Autodesk Inventor part; units mm, degrees
ref_plane "YZ Plane" through (0, 0, 0) normal (1, 0, 0) x (0, 1, 0)
ref_plane "XZ Plane" through (0, 0, 0) normal (0, 1, 0) x (-1, 0, 0)
ref_plane "XY Plane" through (0, 0, 0) normal (0, 0, 1) x (1, 0, 0)
sketch "Sketch1" plane through (0, 0, 0) normal (0, 1, 0) x (-1, 0, 0)
  line L0 (14, 0) -> (0, 0)
  line L1 (0, 0) -> (0, -35.7)
  line L2 (0, -35.7) -> (14, -35.7)
  line L3 (14, -35.7) -> (14, 0)
  circle A0 centre (7, -7) radius 3.25
  circle A1 centre (7, -28.7) radius 3.25
  arc A2 (14, -7) -> (0, -7) centre (7, -7) ccw
  line L4 (14, -35.7) -> (14, -40.7)
  line L5 (14, -40.7) -> (8.75, -40.7)
  line L6 (5.25, -40.7) -> (0, -40.7)
  line L7 (0, -40.7) -> (0, -35.7)
  line L8 (8.75, -40.7) -> (5.25, -40.7)
  line L9 (14, -40.7) -> (46.5741, -73.2741)
  line L10 (46.5741, -73.2741) -> (55.0594, -64.7888)
  line L11 (55.0594, -64.7888) -> (14, -23.7294)
  circle A3 centre (7, -28.7) radius 7
  line L12 (14, -40.7) -> (3.5544, -34.7933)
  point P0 (7, -35.7)
  point P1 (11.375, -40.7)
  point P2 (7, 0)
  point P3 (0, -28.7)
  dimension "d0" = 6.5
  dimension "d1" = 21.7
  dimension "d2" = 7
  dimension "d3" = 7
  dimension "d4" = 14
  dimension "d9" = 5
  dimension "d20" = 12
  dimension "d21" = 135
extrude "Extrusion1" add sketch "Sketch1" along normal blind 4 contours L3 A2 L0 | A2 L1 L0 | A2 L3 A3 L1 | L11 L10 L9 L4 L3 | A3 | L3 L2 A3 | A3 L2 L12 | L4 L12 L2
fillet "Fillet1" radius 5 1 edges at (-14, 2, -40.7)
sketch "Sketch3" plane through (0, 4, 0) normal (0, 1, 0) x (1, 0, 0)
  line L0 (-14, 0) -> (0, 0)
  line L1 (0, 0) -> (0, 28.7)
  arc A0 (0, 28.7) -> (-3.5544, 34.7933) centre (-7, 28.7) ccw
  line L2 (-3.5544, 34.7933) -> (-13.4072, 40.3648)
  arc A1 (-14.4816, 41.1816) -> (-13.4072, 40.3648) centre (-10.946, 44.7171) ccw
  line L3 (-14.4816, 41.1816) -> (-46.5741, 73.2741)
  line L4 (-46.5741, 73.2741) -> (-55.0594, 64.7888)
  line L5 (-55.0594, 64.7888) -> (-14, 23.7294)
  line L6 (-14, 23.7294) -> (-14, 0)
  circle A2 centre (-7, 7) radius 3.25
  circle A3 centre (-7, 28.7) radius 3.25
  circle A4 centre (-7, 28.7) radius 7
  line L7 (-14, 23.7294) -> (-9.3072, 22.0912)
  line L8 (-14, 23.7294) -> (-14, 28.7)
  line L9 (-14.4816, 41.1816) -> (-21.444, 48.144)
  circle A5 centre (-7, 28.7) radius 12.5
  arc A6 (-15.8366, 37.541) -> (-14.4816, 41.1816) centre (-19.1353, 40.8413) ccw
  point P0 (-3.5544, 34.7933)
  point P1 (-11.499, 34.0628)
  point P2 (-3.5544, 34.7933)
  point P3 (-19.4892, 29.2187)
  point P4 (-15.8366, 37.541)
  point P5 (-14.1011, 40.8383)
  point P6 (0, 18.3438)
  point P7 (-12.5691, 39.8909)
  point P8 (-14, 18.3438)
  dimension "d24" = 25
extrude "Extrusion4" add sketch "Sketch3" along normal blind 2.5 contours L5 L4 L3 A6 A5
mirror "Mirror3" about plane through (-34.7643, 6.5, -51.2464) normal (0, 1, 0) of "Extrusion4", "Fillet1", "Extrusion1"
fillet "Fillet3" radius 7 4 edges at (0, 11, 0) (-14, 11, 0) (-14, 2, 0) (0, 2, 0)
properties part number "R2_3DPrint"
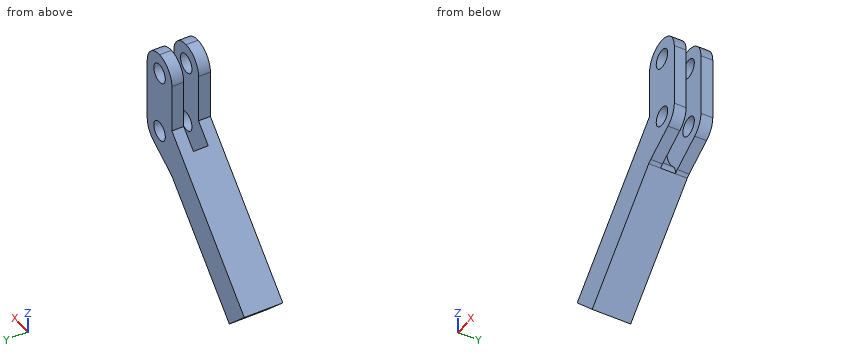
Read the model definition and answer for the solid it produces. Units are mm, in the model's axes. Give positions to 0.01 mm unless a question says otherwise; leave off trailing zeros. Write each loop counter-clockwise with the first axis right and the second up, starting at its lowest first coordinate (ties: lowest second). Pieces come first, ordered by that corner, then holes. Notation, with made-up numbers: (-24.75, -11.75) - (17.25, -11.75) arc R23 ccw to (17.25, 11.25) - close; hole circle Ø9 at (85.5, -1.5). An arc over 180 degrees is marked (long way). Use CSV: the item, a comma, the result in double quotes. Start each with the question number.
(1) Consider line 1 along Z through (x, y) = (-7, 1.7); line 2 along Y through (x, z) = (-13, -13.5); line 3 along X through (y, z) = (10, -4). Determine where each line is inside the solid, lowest interval first.
(2) Find section A-A (z = -18). Give the vertices of the cut face in (x, y), plus the area to 3 significant figures.
(3) Find section D-D (y = 7.25). Give the vertices of the cut face in (x, z), plus the area to 3 significant figures.
(4) Given P1, Ø1.5, axis at x = -21, y = 4.5, coming from the -Z side; P2, Ø4, axis at x = -7, z = -28.7, coming from the -Y side; P3, Ø4.5, axis at y = 1.5, z = -14, coming from the -X side; P4, Ø1, axis at x = -30, y = 5, coming from the +Z side, each flat-ended and moving along its own axis, determine where each tip first touches the part or whether it passes through.
(5) Find section B-B (y = 11.5). Count the separate pieces of the cut face and the enclosed holes in it, plus the area to 3 significant figures.
(6) Find section C-C (x = -5.5). Give the vertices of the cut face in (y, z), plus the area to 3 significant figures.
Findings below:
1,line 1,"-36.74 to -31.95, -25.45 to -10.25, -3.75 to 0"
1,line 2,"0 to 4, 9 to 13"
1,line 3,"-13.32 to -8.25, -5.75 to -0.68"
2,outline,"(-14, 0) - (0, 0) - (0, 4) - (-14, 4) - close; (-14, 9) - (0, 9) - (0, 13) - (-14, 13) - close"
2,area,"112 mm2"
3,outline,"(-55.06, -64.79) - (-46.57, -73.27) - (-14.48, -41.18) arc R4.67 ccw to (-15.84, -37.54) arc R12.5 cw to (-19.49, -29.22) - close"
3,area,"571 mm2"
4,P1,"z = -48.45"
4,P2,"through"
4,P3,"x = -14"
4,P4,"z = -39.23"
5,separate pieces,"1"
5,enclosed holes,"2"
5,area,"1,050 mm2"
6,outline,"(0, -35.89) - (4, -35.89) - (4, -31.58) - (0, -31.58) - close; (0, -25.82) - (4, -25.82) - (4, -9.88) - (0, -9.88) - close; (0, -4.12) - (4, -4.12) - (4, -0.16) - (0, -0.16) - close; (9, -35.89) - (13, -35.89) - (13, -31.58) - (9, -31.58) - close; (9, -25.82) - (13, -25.82) - (13, -9.88) - (9, -9.88) - close; (9, -4.12) - (13, -4.12) - (13, -0.16) - (9, -0.16) - close"
6,area,"194 mm2"
